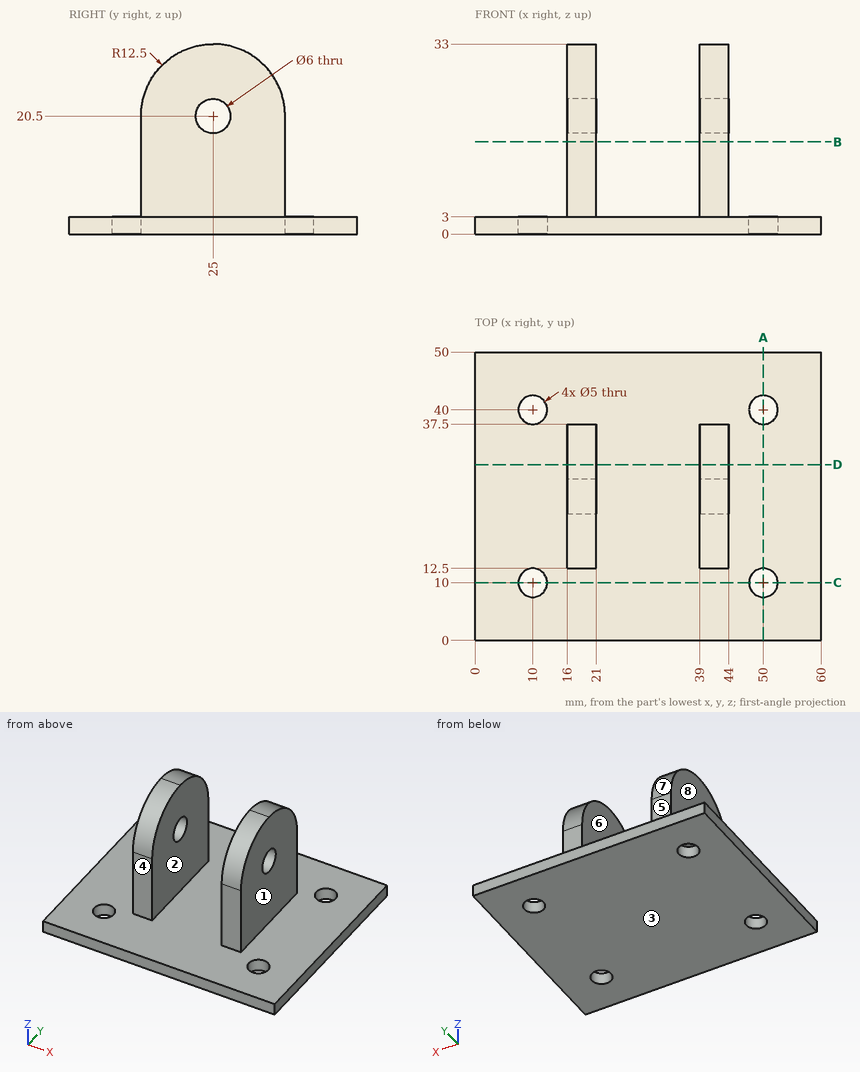
Here's the drawing with two shaded views (mm, measured from the low corner). I have some questions. A direction names the side the tool comes from. Give positions to 0.01 mm unless a question says otherwise; leave off trailing zeros. Write each loop counter-clockwise with the first axis right and the second up, starting at its lowest first coordinate (ties: lowest second). Pieces come first, ordered by that corner, then holes. Notation, with made-up numbers: (74, 42) - (112, 42) arc R27 ccw to (112, 63) - close; hole circle Ø9 at (40.25, 5.25). An arc over 180 degrees is marked (long way). Write item = value, one per line. Start each with the question number.
1. On a 3-axis mill with a long thin cutter (end or side, diameter ignored), from which of +Z, -Z, +X, -X, +Y, -Y can I reach the whole of each face in a straight line? I mean the marked faces 1, 2, 3, 4 and 5. Say none if no direction works.
2. Please list where these lines run through material, in increasing order: line 1 (Y direction, x = 10, z = 2); line 2 (X direction, y = 30, z = 15.5); line 3 (Z direction, x = 11.5, y = 32).
3. Thinking about a two-plate mould opening in X: for the marked faces 6, 7 and 8, which applies, released by +X, released by -X, zero draft, split by the parting line, or undercut?
4. For pin 1 (4 mm diameter, centred on x = 40, z = 9, fed in from +Y); pin 2 (7.5 mm diameter, centred on y = 24.5, z = 22.5, fed in from +X); pin 3 (6 mm diameter, centred on x = 35, z = 26.5, fed in from -Y); pin 4 (10 mm diameter, centred on y = 19, z = 26.5, fed in from -X), each with a flat end and sliding along its axis, tell me the tip position at first contact or that it passes through.
5. Imagine slicing it at C-C (y = 10). Please give me the cut outline in (x, z), and give its area (3 significant figures).
6. Imagine slicing it at B-B (z = 16). Please give me the cut outline in (x, y), and give its area (3 significant figures).
7. Imagine slicing it at D-D (y = 30.5). Please give me the cut outline in (x, z) (3 decimals).
8. Imagine slicing it at A-A (x = 50). Please give me the cut outline in (y, z), and give its area (3 significant figures).
Worked answers:
q1.face_1 = +Z, +X, +Y, -Y
q1.face_2 = +Z, +Y, -Y
q1.face_3 = -Z, +X, -X, +Y, -Y
q1.face_4 = +Z, +X, -X, -Y
q1.face_5 = +Z, +X, -X, +Y
q2.line_1 = 0 to 7.5, 12.5 to 37.5, 42.5 to 50
q2.line_2 = 16 to 21, 39 to 44
q2.line_3 = 0 to 3
q3.face_6 = undercut
q3.face_7 = zero draft
q3.face_8 = released by -X
q4.pin_1 = 37.5
q4.pin_2 = 44
q4.pin_3 = through
q4.pin_4 = 16
q5.outline = (0, 0) - (7.5, 0) - (7.5, 3) - (0, 3) - close; (12.5, 0) - (47.5, 0) - (47.5, 3) - (12.5, 3) - close; (52.5, 0) - (60, 0) - (60, 3) - (52.5, 3) - close
q5.area = 150 mm2
q6.outline = (16, 12.5) - (21, 12.5) - (21, 37.5) - (16, 37.5) - close; (39, 12.5) - (44, 12.5) - (44, 37.5) - (39, 37.5) - close
q6.area = 250 mm2
q7.outline = (0, 0) - (60, 0) - (60, 3) - (44, 3) - (44, 31.725) - (39, 31.725) - (39, 3) - (21, 3) - (21, 31.725) - (16, 31.725) - (16, 3) - (0, 3) - close
q8.outline = (0, 0) - (7.5, 0) - (7.5, 3) - (0, 3) - close; (12.5, 0) - (37.5, 0) - (37.5, 3) - (12.5, 3) - close; (42.5, 0) - (50, 0) - (50, 3) - (42.5, 3) - close
q8.area = 120 mm2
